Input: part model. Units: mm. Frame: model coordinates. Give positions to 0.01 mm unless a question says otherwise; leave off trailing zeros. Write each loop counter-clockwise with the first axis right and the second up, starting at its lowest first coordinate (ties: lowest second). Pieces come first, ordered by that corner, then holes. Notation, with made-up numbers: (-9, -25) - (5, -25) arc R14 cw to (5, -21) - close; hole circle Ø4 at (82, 78). An arc over 180 degrees is marked (long way). Answer as CSV lines item,"result".
```python
from build123d import *

# Parameters (mm, degrees)
SKETCH1_R           = 2.6
SKETCH1_W           = 34.8
SKETCH1_H           = 36.503761473
BOSS_EXTRUDE1_DEPTH = 3
CHAMFER1_SIZE       = 3


with BuildPart() as part:
    # Sketch1 → Boss-Extrude1 (new body)
    with BuildSketch(Plane(origin=(0, 0, 0), x_dir=(1, 0, 0), z_dir=(0, 1, 0))):
        Polygon((-36.075215726, -21.465620287), (-18.775215726, -21.465620287), (22.024784274, -21.465620287), (39.324784274, -21.465620287), (39.324784274, 21.038141186), (22.024784274, 21.038141186), (-18.775215726, 21.038141186), (-36.075215726, 21.038141186), align=None)
        with Locations(Location((-27.925215726, -10.265620287, 0), (0, 0, 270))):
            Circle(SKETCH1_R, mode=Mode.SUBTRACT)
        with Locations(Location((31.174784274, -10.161858814, 0), (0, 0, 270))):
            Circle(SKETCH1_R, mode=Mode.SUBTRACT)
        with Locations(Location((-27.925215726, 9.734379713, 0), (0, 0, 270))):
            Circle(SKETCH1_R, mode=Mode.SUBTRACT)
        with Locations((1.624784274, -0.21373955)):
            Rectangle(SKETCH1_W, SKETCH1_H, mode=Mode.SUBTRACT)
        with Locations(Location((31.174784274, 9.838141186, 0), (0, 0, 270))):
            Circle(SKETCH1_R, mode=Mode.SUBTRACT)
    extrude(amount=BOSS_EXTRUDE1_DEPTH)

    # Chamfer1
    chamfer1_edges = [part.edges().sort_by_distance(p)[0] for p in [
        (-36.075215726, 1.5, 21.465620287),
        (-36.075215726, 1.5, -21.038141186),
        (39.324784274, 1.5, -21.038141186),
        (39.324784274, 1.5, 21.465620287),
    ]]
    chamfer(chamfer1_edges, length=CHAMFER1_SIZE)


solid = part.part
```
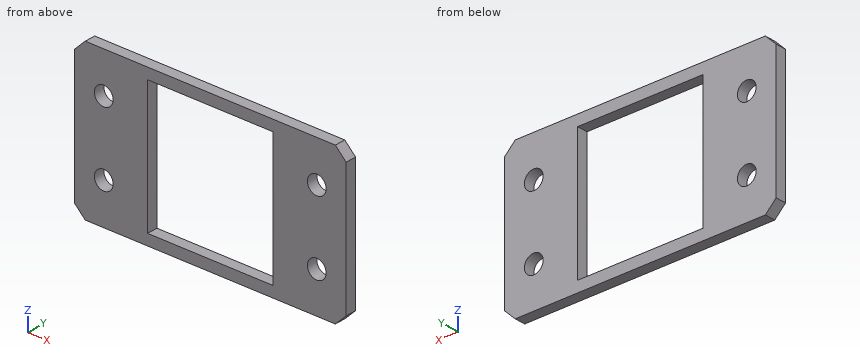
Item 1: Cut plane B-B on z = -16.5. Return the cut outline in (x, y), plus the area to 3 significant figures.
The answers:
outline,"(-36.08, 0) - (-15.78, 0) - (-15.78, 3) - (-36.08, 3) - close; (19.02, 0) - (39.32, 0) - (39.32, 3) - (19.02, 3) - close"
area,"122 mm²"
Item 2: Ray query, line 1 (X direction, y = 2.05, z = 2); line 2 (Z direction, x = -11.5, y = 0.75); line 3 (Z direction, x = 30.5, y = 1.2). Return the intervals inside material, ascending. Write a range as from..to.
The answers:
line 1,"-36.08..-15.78, 19.02..39.32"
line 2,"-21.04..-18.04, 18.47..21.47"
line 3,"-21.04..-12.35, -7.33..7.65, 12.67..21.47"
Item 3: Cut plane A-A on x = 2. Return the cut outline in (y, z), plus the area to 3 significant figures.
The answers:
outline,"(0, -21.04) - (3, -21.04) - (3, -18.04) - (0, -18.04) - close; (0, 18.47) - (3, 18.47) - (3, 21.47) - (0, 21.47) - close"
area,"18.0 mm²"
Item 4: Cut plane C-C on y = 1.15. Return the cut outline in (x, z), plus the area to 3 significant figures.
The answers:
outline,"(-36.08, -18.04) - (-33.08, -21.04) - (36.32, -21.04) - (39.32, -18.04) - (39.32, 18.47) - (36.32, 21.47) - (-33.08, 21.47) - (-36.08, 18.47) - close; hole circle Ø5.2 at (-27.93, -9.73); hole circle Ø5.2 at (-27.93, 10.27); hole (-15.78, -18.04) - (19.02, -18.04) - (19.02, 18.47) - (-15.78, 18.47) - close; hole circle Ø5.2 at (31.17, -9.84); hole circle Ø5.2 at (31.17, 10.16)"
area,"1,830 mm²"
